Can you work these out from the drawing? Everything is in mm from the part's minimum corner. Coordinates: 2 decimals unless noted, no trailing zeros. Loops run counter-clockwise (first coordinate to the right, second up) from the corner with the lowest first, then second, coordinate; pieces in that order, holes last. Notation, with made-up numbers: (3.25, 15) -> (16.25, 15) arc R14 ccw to (16.25, 39) -> close; hole circle Ø4 at (-26, 44). An arc over 180 degrees is marked (long way). Put each result on its own line as item: value. Start each with the question number.
Item 1: Please list where this line runs through material, in increasing order: L1, parallel to X at y = 24.5, z = 15.75. Write a range as from..to.
Item 2: If we section it at A-A on z = 12.5: Please give me the cut outline in (x, y).
Item 3: Will these pins go through, and if not, where does the flat tip stop? P1, Ø3, axis at y = 22.5, z = 5.5, coming from the -X side; P2, Ø1, axis at x = 132.5, z = 5.5, coming from the -Y side; P3, Ø4.5, axis at y = 23, z = 13.5, coming from the +X side.
Item 4: If we section it at B-B on y = 23: Please give me the cut outline in (x, z).
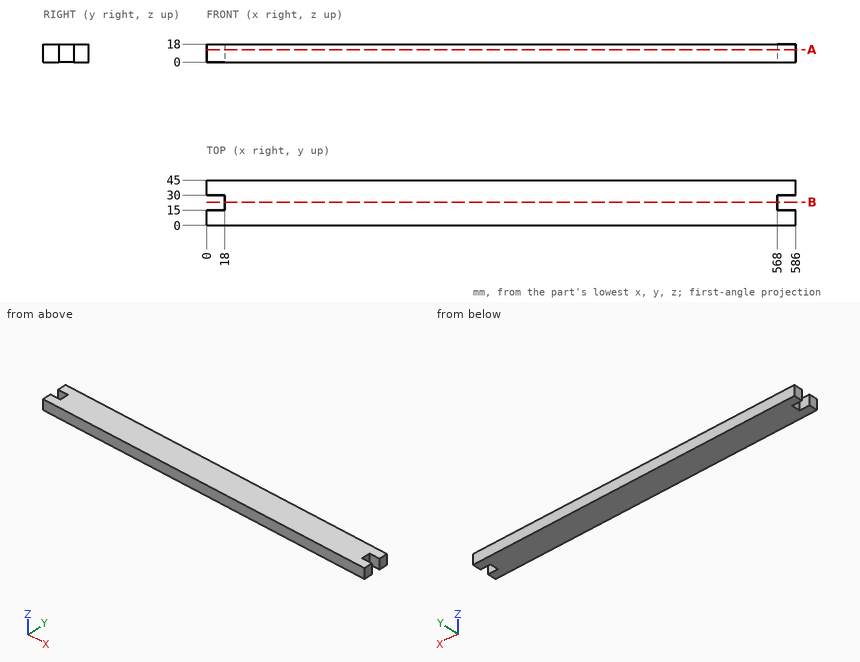
Solutions:
1. L1: 18..568
2. outline: (0, 0) -> (586, 0) -> (586, 15) -> (568, 15) -> (568, 30) -> (586, 30) -> (586, 45) -> (0, 45) -> (0, 30) -> (18, 30) -> (18, 15) -> (0, 15) -> close
3. P1: x = 18
3. P2: y = 0
3. P3: x = 568
4. outline: (18, 0) -> (568, 0) -> (568, 18) -> (18, 18) -> close
